Autodesk Inventor part; units mm, degrees
ref_plane "YZ Plane" through (0, 0, 0) normal (1, 0, 0) x (0, 1, 0)
ref_plane "XZ Plane" through (0, 0, 0) normal (0, 1, 0) x (-1, 0, 0)
ref_plane "XY Plane" through (0, 0, 0) normal (0, 0, 1) x (1, 0, 0)
sketch "Boceto1" plane through (0, 0, 0) normal (0, 0, 1) x (1, 0, 0)
  line L0 (0, 0) -> (88, 0)
  line L1 (88, 0) -> (88, 88)
  line L2 (88, 88) -> (79.3, 88)
  line L3 (79.3, 88) -> (79.3, 8.7)
  line L4 (79.3, 8.7) -> (0, 8.7)
  line L5 (0, 8.7) -> (0, 0)
  dimension "d0" = 8.7
  dimension "d1" = 8.7
  dimension "d2" = 88
  dimension "d3" = 88
extrude "Extrusión1" add sketch "Boceto1" along normal blind 43
sketch "Boceto2" plane through (0, 0, 0) normal (0, 0, -1) x (-1, 0, 0)
  line L0 (-88, 88) -> (-79.3, 88)
  line L1 (-79.3, 88) -> (-71.8, 88)
  line L2 (-71.8, 88) -> (-71.8, 79)
  line L3 (-71.8, 79) -> (-9, 16.2)
  line L4 (-9, 16.2) -> (0, 16.2)
  line L5 (-79.3, 88) -> (-79.3, 8.7)
  line L6 (-79.3, 8.7) -> (0, 8.7)
  line L7 (0, 8.7) -> (0, 16.2)
  point P0 (0, 0)
  dimension "d6" = 7.5
  dimension "d7" = 7.5
  dimension "d8" = 9
  dimension "d9" = 9
extrude "Extrusión2" add sketch "Boceto2" against normal blind 5
sketch "Boceto3" plane through (79.3, 8.7, 43) normal (-1, 0, 0) x (0, 0, 1)
  line L0 (-19, 36.55) -> (-19, 14.65) construction
  line L1 (-24.65, 36.55) -> (-24.65, 14.65)
  line L2 (-13.35, 14.65) -> (-13.35, 36.55)
  arc A0 (-13.35, 36.55) -> (-24.65, 36.55) centre (-19, 36.55) ccw
  arc A1 (-24.65, 14.65) -> (-13.35, 14.65) centre (-19, 14.65) ccw
  circle A2 centre (-19, 59.3) radius 5.65
  line L3 (-38, 79.3) -> (0, 79.3)
  line L4 (-38, 0) -> (0, 0)
  point P0 (-43, -8.7)
  point P1 (-19, 25.6)
  point P2 (-19, 79.3)
  point P3 (-19, 9)
  point P4 (-19, 42.2)
  dimension "d12" = 11.3
  dimension "d13" = 20
  dimension "d14" = 11.3
  dimension "d15" = 33.2
  dimension "d16" = 9
extrude "Extrusión3" cut sketch "Boceto3" against normal through all
sketch "Boceto4" plane through (0, 8.7, 43) normal (0, 1, 0) x (1, 0, 0)
  circle A0 centre (20, 19) radius 5.65
  line L0 (64.65, 19) -> (42.75, 19) construction
  line L1 (64.65, 24.65) -> (42.75, 24.65)
  line L2 (42.75, 13.35) -> (64.65, 13.35)
  arc A1 (64.65, 13.35) -> (64.65, 24.65) centre (64.65, 19) ccw
  arc A2 (42.75, 24.65) -> (42.75, 13.35) centre (42.75, 19) ccw
  line L3 (0, 38) -> (0, 0)
  line L4 (79.3, 38) -> (79.3, 0)
  point P0 (0, 43)
  point P1 (53.7, 19)
  point P2 (0, 19)
  point P3 (70.3, 19)
  point P4 (37.1, 19)
  dimension "d19" = 11.3
  dimension "d20" = 11.3
  dimension "d21" = 9
  dimension "d22" = 33.2
  dimension "d23" = 20
extrude "Extrusión4" cut sketch "Boceto4" against normal through all
equation "\"d1\" = d0"
equation "\"d3\" = d2"
equation "\"d7\" = d6"
equation "\"d14\" = d12"
equation "\"d20\" = d19"
properties part number "escuadra grande"
CAD build for the part. Positions are in the model's coordinates, mm. A direction names the side the tool comes from. Round coordinates to 2 decimals unless told otherwise and drop trailing zeros. Write each loop counter-clockwise with the first axis right and the second up, starting at its lowest first coordinate (ties: lowest second). Pieces come first, ordered by that corner, then holes. Notation, with made-up numbers: (44.5, 72) -> (100.5, 72) arc R18 cw to (100.5, 100) -> close; hole circle Ø4 at (71.5, 56.25). An arc over 180 degrees is marked (long way). Answer in a Markdown table with one row per item. Add a question column.
Item 1: Saw through at B-B, the plane z = 24. Write the cut outline in (x, y).
Item 2: Drop flat-ended pins along their axis: pin 1 Ø13 at (y, z) = (68, 24) entering from -X; pin 2 Ø4 at (y, z) = (81.5, 3) entering from -X; pin 3 Ø6 at (x, z) = (71.5, 25.5) entering from +Y. Give the stop position or say it passes through.
Item 3: Saw through at D-D, the plane x = 80.5. Write the cut outline in (y, z).
Item 4: Drill centre lines: line 1 (X direction, y = 4.75, z = 24); line 2 (Y direction, x = 86.25, z = 24); line 3 (Z direction, x = 62, y = 32). Where is each one in solid material? Low to high. Write a range as from..to.
Item 5: Which spindle directions (+Z, -Z, +X, -X, +Y, -Y) get a long thin tool onto all of the face, cutting with end or side? Do faces 4 (the face through (37.1, 4.4, 23.9)), 5 (the face through (79.3, 58, 24)), 6 (the face through (71.8, 84, 2)), 7 (the face through (83.6, 50.9, 24.1)). Say none if no direction does.
Item 6: Mould opens along Y. For faces 1 (the face through (84, 34, 29.65)), 2 (the face through (58, 31, 5)), 3 (the face through (40.8, 48, 2.5)) say: pulls with the +Y half, pulls with the -Y half, needs draft (parallel to the pull), parting line crosses it, or undercut.
Item 7: Saw through at C-C, the plane y = 28. Write the cut outline in (x, z), then the cut area to 3 significant figures.
Item 8: Saw through at A-A, the plane x = 20. Write the cut outline in (y, z), then the cut area to 3 significant figures.
Findings below:
| question | item | result |
|---|---|---|
| 1 | outline | (0, 0) -> (14.35, 0) -> (14.35, 8.7) -> (0, 8.7) -> close; (25.65, 0) -> (37.1, 0) -> (37.1, 8.7) -> (25.65, 8.7) -> close; (70.3, 0) -> (88, 0) -> (88, 17.7) -> (79.3, 17.7) -> (79.3, 8.7) -> (70.3, 8.7) -> close; (79.3, 50.9) -> (88, 50.9) -> (88, 62.35) -> (79.3, 62.35) -> close; (79.3, 73.65) -> (88, 73.65) -> (88, 88) -> (79.3, 88) -> close |
| 2 | pin 1 | stops at x = 79.3 |
| 2 | pin 2 | stops at x = 71.8 |
| 2 | pin 3 | stops at y = 8.7 |
| 3 | outline | (0, 0) -> (88, 0) -> (88, 43) -> (0, 43) -> close; hole (23.35, 18.35) -> (45.25, 18.35) arc R5.65 ccw to (45.25, 29.65) -> (23.35, 29.65) arc R5.65 ccw to start; hole circle Ø11.3 at (68, 24) |
| 4 | line 1 | x = 0..14.35, 25.65..37.1, 70.3..88 |
| 4 | line 2 | y = 0..17.7, 50.9..62.35, 73.65..88 |
| 4 | line 3 | z = 0..5 |
| 5 | face 4 | +Y, -Y |
| 5 | face 5 | +Z, -X, +Y |
| 5 | face 6 | +Z, -Z, -X, +Y |
| 5 | face 7 | +X, -X |
| 6 | face 1 | undercut |
| 6 | face 2 | needs draft |
| 6 | face 3 | pulls with the +Y half |
| 7 | outline | (20.8, 0) -> (88, 0) -> (88, 18.35) -> (79.3, 18.35) -> (79.3, 5) -> (20.8, 5) -> close; (79.3, 29.65) -> (88, 29.65) -> (88, 43) -> (79.3, 43) -> close |
| 7 | area | 568 mm^2 |
| 8 | outline | (0, 0) -> (27.2, 0) -> (27.2, 5) -> (8.7, 5) -> (8.7, 18.35) -> (0, 18.35) -> close; (0, 29.65) -> (8.7, 29.65) -> (8.7, 43) -> (0, 43) -> close |
| 8 | area | 368 mm^2 |
